Geometry check sheet. Reference: the model listing, model coordinates, mm. A direction names the side the tool comes from. Round coordinates to 2 decimals unless told otherwise and drop trailing zeros. Write each loop counter-clockwise with the first axis right and the second up, starting at its lowest first coordinate (ties: lowest second). Pieces come first, ordered by that corner, then holes. Notation, with made-up numbers: (-28, 36.25) - (23, 36.25) arc R13 cw to (23, 61.25) - close; hole circle Ø5 at (-21.75, 59.5). An arc over 180 degrees is marked (long way). Return JSON: item names as keys, results as strings.
```python
from build123d import *

# Parameters (mm, degrees)
SKETCH1_W                    = 8.5
SKETCH1_H                    = 14.5
CUT_EXTRUDE1_REACH           = 2.1
CUT_EXTRUDE2_REACH           = 2.1
CUT_EXTRUDE3_REACH           = 2.1
CUT_EXTRUDE4_REACH           = 2.1
F_2_0_2_DIAMETER_HOLE1_D     = 2
F_2_0_2_DIAMETER_HOLE1_DEPTH = 3
F_2_0_2_DIAMETER_HOLE2_D     = 3.2
F_2_0_2_DIAMETER_HOLE2_DEPTH = 3.5
F_2_0_2_DIAMETER_HOLE3_D     = 2
F_2_0_2_DIAMETER_HOLE3_DEPTH = 3
F_2_0_2_DIAMETER_HOLE4_D     = 3.2
F_2_0_2_DIAMETER_HOLE4_DEPTH = 3.5


with BuildPart() as part:
    # Sketch1 → Revolve1 (revolve)
    with BuildSketch(Plane(origin=(0, 0, 0), x_dir=(-1, 0, 0), z_dir=(0, 0, -1))):
        with Locations((-4.25, 7.25)):
            Rectangle(SKETCH1_W, SKETCH1_H)
    revolve(axis=Axis((0, 0, 0), (0, 1, 0)))

    # Sketch2 → Cut-Extrude1 (cut, up to next)
    with BuildSketch(Plane(origin=(-8.4, 0, 0), x_dir=(0, 0, -1), z_dir=(1, 0, 0)), mode=Mode.PRIVATE) as cut_extrude1_sk1:
        Polygon((0.9, 13.234042555), (0.9, 13.297872335), (0.649999993, 13.297872335), (0.649999993, 13.553191453), (0.587500007, 13.553191453), (0.587500007, 13.297872335), (0.3375, 13.297872335), (0.3375, 13.234042555), (0.587500007, 13.234042555), (0.587500007, 12.978723392), (0.649999993, 12.978723392), (0.649999993, 13.234042555), align=None)
    cut_extrude1_tool1 = extrude(cut_extrude1_sk1.sketch, amount=-CUT_EXTRUDE1_REACH, mode=Mode.PRIVATE) & part.part
    add(cut_extrude1_tool1.solids().sort_by_distance((-8.4, 13.265957, -0.61875))[0], mode=Mode.SUBTRACT)

    # Sketch3 → Cut-Extrude2 (cut, up to next)
    with BuildSketch(Plane.XY.offset(-8.4), mode=Mode.PRIVATE) as cut_extrude2_sk1:
        Polygon((1, 13.234042555), (1, 13.297872335), (0.749999993, 13.297872335), (0.749999993, 13.553191453), (0.687500007, 13.553191453), (0.687500007, 13.297872335), (0.4375, 13.297872335), (0.4375, 13.234042555), (0.687500007, 13.234042555), (0.687500007, 12.978723392), (0.749999993, 12.978723392), (0.749999993, 13.234042555), align=None)
    cut_extrude2_tool1 = extrude(cut_extrude2_sk1.sketch, amount=-CUT_EXTRUDE2_REACH, mode=Mode.PRIVATE) & part.part
    add(cut_extrude2_tool1.solids().sort_by_distance((0.71875, 13.265957, -8.4))[0], mode=Mode.SUBTRACT)

    # Sketch4 → Cut-Extrude3 (cut, up to next)
    with BuildSketch(Plane.XY.offset(-8.4), mode=Mode.PRIVATE) as cut_extrude3_sk1:
        Polygon((-0.875, 12.5), (-0.43749997, 13.106382996), (-3e-08, 12.5), (0.18749997, 12.5), (-0.34374997, 13.265957445), (0.18749997, 14), (-3e-08, 14), (-0.43749997, 13.393617004), (-0.875, 14), (-1.0625, 14), (-0.53125006, 13.265957445), (-1.0625, 12.5), align=None)
    cut_extrude3_tool1 = extrude(cut_extrude3_sk1.sketch, amount=-CUT_EXTRUDE3_REACH, mode=Mode.PRIVATE) & part.part
    add(cut_extrude3_tool1.solids().sort_by_distance((-0.4375, 13.242259, -8.4))[0], mode=Mode.SUBTRACT)

    # Sketch5 → Cut-Extrude4 (cut, up to next)
    with BuildSketch(Plane(origin=(-8.4, 0, 0), x_dir=(0, 0, -1), z_dir=(1, 0, 0)), mode=Mode.PRIVATE) as cut_extrude4_sk1:
        Polygon((-1.10000006, 14), (-0.6, 13.265957445), (-0.6, 12.5), (-0.4125, 12.5), (-0.4125, 13.265957445), (0.08749997, 14), (-0.10000003, 14), (-0.50625, 13.393617004), (-0.91250006, 14), align=None)
    cut_extrude4_tool1 = extrude(cut_extrude4_sk1.sketch, amount=-CUT_EXTRUDE4_REACH, mode=Mode.PRIVATE) & part.part
    add(cut_extrude4_tool1.solids().sort_by_distance((-8.4, 13.37564, 0.50625))[0], mode=Mode.SUBTRACT)

    # Sketch6 → Revolve2 (revolve)
    with BuildSketch(Plane(origin=(0, 2.49, 0), x_dir=(1, 0, 0), z_dir=(0, 1, 0))):
        Polygon((-6.537367948, -13.647813756), (-4.635254916, -14.265847744), (-2.552899345, -7.857016287), (-4.455012378, -7.238982298), align=None)
    revolve(axis=Axis((-4.635254916, 2.49, 14.265847744), (0.309016994, 0, -0.951056516)))

    # Ø2.0 (2) Diameter Hole1
    with Locations(Plane(origin=(0, 0, 0), x_dir=(-1, 0, 0), z_dir=(0, -1, 0))):
        with Locations((1.08530111, 6.155048456), (-5.87307888, -2.137625896)):
            Hole(F_2_0_2_DIAMETER_HOLE1_D / 2, depth=F_2_0_2_DIAMETER_HOLE1_DEPTH)

    # Ø2.0 (2) Diameter Hole2
    with Locations(Plane(origin=(0, 0, 0), x_dir=(-1, 0, 0), z_dir=(0, -1, 0))):
        with Locations((6.226216863, -0.544723392), (-3.584852727, -5.119700277), (-2.641364136, 5.664423669)):
            Hole(F_2_0_2_DIAMETER_HOLE2_D / 2, depth=F_2_0_2_DIAMETER_HOLE2_DEPTH)

    # Ø2.0 (2) Diameter Hole3
    with Locations(Plane(origin=(0, 14.5, 0), x_dir=(1, 0, 0), z_dir=(0, 1, 0))):
        with Locations((0, 6.25), (-5.412658774, -3.125)):
            Hole(F_2_0_2_DIAMETER_HOLE3_D / 2, depth=F_2_0_2_DIAMETER_HOLE3_DEPTH)

    # Ø2.0 (2) Diameter Hole4
    with Locations(Plane(origin=(0, 14.5, 0), x_dir=(1, 0, 0), z_dir=(0, 1, 0))):
        with Locations((0, -6.25), (5.412658774, 3.125), (-5.412658774, 3.125)):
            Hole(F_2_0_2_DIAMETER_HOLE4_D / 2, depth=F_2_0_2_DIAMETER_HOLE4_DEPTH)


solid = part.part
```
(1) Section check B-B, the plane z = 6.25. Enter the section's corners in (x, y).
Response values:
{"outline": "(-5.76, 0) - (2.45, 0) - (2.45, 3.5) - (4.72, 3.5) - (4.72, 0) - (5.76, 0) - (5.76, 14.5) - (1.6, 14.5) - (1.6, 11) - (-1.6, 11) - (-1.6, 14.5) - (-5.76, 14.5) - close"}
(2) Material ranges on line 1 along Z through (x, y) = (0, 13.4); line 2 along X through (y, z) = (13, 5.75); line 3 along Y through (x, z) = (-5.75, 11.75), recorded low to high. Write a range as [from, to].
Response values:
{"line 1": "z = [-8.5, -7.25], [-5.25, 4.65], [7.85, 8.5]", "line 2": "x = [-6.26, -1.52], [1.52, 6.26]", "line 3": "y = [1.7, 3.28]"}
(3) Section check C-C, the plane y = 9. Enter the section's corners in (x, z), plus the area to 3 significant figures.
Response values:
{"outline": "circle Ø17 at (0, 0)", "area": "227 mm^2"}
(4) Gauge pin test, flat ends, axial feed: pin 1 (4 mm diameter, centred on x = -6.5, y = 4.5, fed in from +Z); pin 2 (3 mm diameter, centred on x = -6.23, z = 0.54, fed in from -Y); pin 3 (6 mm diameter, centred on x = -6.5, y = 12, fed in from -Z); pin 4 (8 mm diameter, centred on x = -1.5, y = 3, fed in from +Z). Record the tip position at first contact, or that the pin passes through.
Response values:
{"pin 1": "stops at z = 14.31", "pin 2": "stops at y = 3.5", "pin 3": "stops at z = -7.75", "pin 4": "stops at z = 14.88"}
(5) Section check A-A, the plane y = 1.75. Enter the section's corners in (x, z).
Response values:
{"outline": "(-6.4, 13.69) - (-4.33, 7.31) arc R8.5 ccw (long way) to (-0.8, 8.46) - (-2.87, 14.84) - close; hole circle Ø3.2 at (-6.23, 0.54); hole circle Ø2 at (-1.09, -6.16); hole circle Ø3.2 at (2.64, -5.66); hole circle Ø3.2 at (3.58, 5.12); hole circle Ø2 at (5.87, 2.14)"}
(6) Release check for a two-part mould opening along X. For faces 1 (the face through (-5, 11, -3)), 2 (the face through (0, 14.5, 0)) record: pulls with the +X half, pulls with the -X half, needs draft (parallel to the pull), parting line crosses it, or undercut.
Response values:
{"face 1": "undercut", "face 2": "needs draft"}
(7) Access from +Z, -Z, +X, -X, +Y, -Y to the whole of each face (thin tool, end or side, straight path). Record for faces 3 (the face through (6.68, 12.73, -2.15)), 4 (the face through (-4.7, 1.77, 0.06)).
Response values:
{"face 3": "+Y", "face 4": "-Y"}
